Design review of the part shown in the three views and the two pictorial views. Dimensions are in mm from the part's minimum x, y and z. A direction names the side the tool comes from. Give positions to 0.01 mm unless a question says otherwise; leave off trailing zeros. Loops run counter-clockwise (first coordinate to the right, second up) from the corner with the lowest first, then second, coordinate; pieces in that order, holes last. Notation, with made-up numbers: (83, 84.25) - (114, 84.25) arc R33 ccw to (114, 115.25) - close; hole circle Ø3 at (-34.75, 79). An arc over 180 degrees is marked (long way). Return JSON: item names as keys, results as strings. Group by question number.
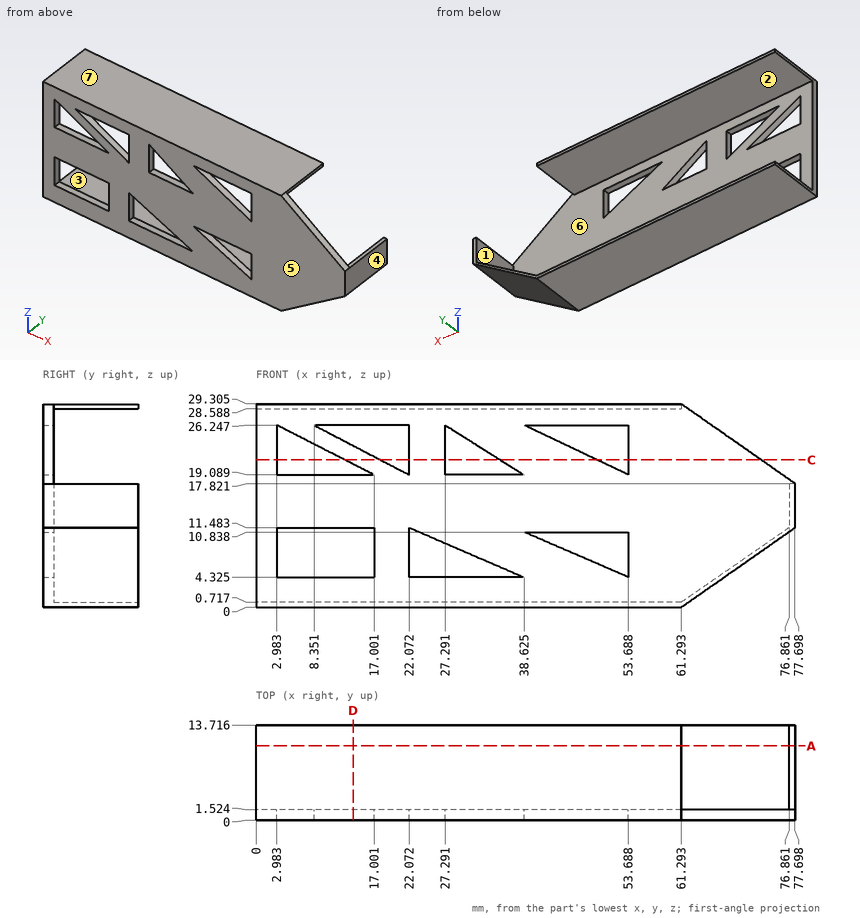
Item 1: For L1, parallel to Z at x = 18.5, y = 6.5 (1 decimal); L2, parallel to Z at x = 43.5, y = 1.25 (1 decimal); L3, parallel to X at y = 0.5, z = 6.75 (1 decimal), list the stretches that pass through material, from the lowest coordinate up. Write a range as from..to.
Item 2: Take a section at D-D (x = 14). State the section outline as (y, z) points (1 decimal).
Item 3: Tool access review of the marked faces 1, 2, 3 and 4: name each direction out of +Z, -Z, +X, -X, +Y, -Y from which nothing blocks a thin tool from reaching the whole face with its end or side.
Item 4: Take a section at C-C (z = 21.25). State the section outline as (x, y) points.
Item 5: Take a section at A-A (y = 10.75). State the section outline as (x, z) points (1 decimal).
Item 6: Mouldability with a two-part tool opening along Z and no side actions: class the marked faces 5, 6 and 7 as +Z half, -Z half, draft (parallel to the pull), parting line (faces both ways), or undercut.
Item 7: For P1, Ø1.2, axis at y = 1, z = 23.5, coming from the +X side (1 decimal); P2, Ø0.6, axis at y = 5, z = 29, coming from the +X side; P3, Ø6, axis at y = 10.5, z = 24.5, coming from the -X side; P4, Ø4, axis at y = 6, z = 6.5, coming from the -X side (1 decimal), all flat-tipped, find the tip position at first contact; note any pin that passes through.
Check sheet entries:
{
 "1": {"L1": "z = 0..0.7, 28.6..29.3", "L2": "z = 0..8.7, 10.8..23.9, 26.2..29.3", "L3": "x = 0..3, 17..22.1, 33..48.1, 53.7..70.9"},
 "2": {"outline": "(0, 0) - (13.7, 0) - (13.7, 0.7) - (1.5, 0.7) - (1.5, 4.3) - (0, 4.3) - close; (0, 11.5) - (1.5, 11.5) - (1.5, 19.1) - (0, 19.1) - close; (0, 20.6) - (1.5, 20.6) - (1.5, 23.3) - (0, 23.3) - close; (0, 26.2) - (1.5, 26.2) - (1.5, 28.6) - (13.7, 28.6) - (13.7, 29.3) - (0, 29.3) - close"},
 "3": {"face 1": "+Z, -X, +Y", "face 2": "+X, -X, +Y", "face 3": "-X, +Y", "face 4": "+Z, -Z, +X, +Y, -Y"},
 "4": {"outline": "(0, 0) - (2.98, 0) - (2.98, 1.52) - (0, 1.52) - close; (12.77, 0) - (17.93, 0) - (17.93, 1.52) - (12.77, 1.52) - close; (22.07, 0) - (27.29, 0) - (27.29, 1.52) - (22.07, 1.52) - close; (35.2, 0) - (49.14, 0) - (49.14, 1.52) - (35.2, 1.52) - close; (53.69, 0) - (72.8, 0) - (72.8, 1.52) - (53.69, 1.52) - close"},
 "5": {"outline": "(0, 0) - (61.3, 0) - (77.7, 11.5) - (77.7, 17.8) - (76.9, 17.8) - (76.9, 11.5) - (61.3, 0.7) - (0, 0.7) - close; (0, 28.6) - (61.3, 28.6) - (61.3, 29.3) - (0, 29.3) - close"},
 "6": {"face 5": "draft", "face 6": "undercut", "face 7": "+Z half"},
 "7": {"P1": "stops at x = 70.4", "P2": "stops at x = 61.29", "P3": "passes through", "P4": "stops at x = 66.8"}
}
